Read the model definition and answer for the solid it produces. Units are mm, in the model's axes. Give positions to 0.01 mm unless a question says otherwise; leave off trailing zeros. Write each question's results on one line, items separated by ' | '. Start each with the question number.
Item 1: Determine the mould class of faces 1 (the cylindrical face through (-9.29, 3.13, 27.62)), 2 (the flat face through (0, 6.35, -1)), 3 (the cylindrical face through (-23.208, 3.219, 58.415)) for opening direction X: +X half, -X half, draft (parallel to the pull), parting line (faces both ways), or undercut.
Item 2: Section A-A on y = 4 is taken. State how many separate pieces and enclosed holes the cut face has, and give its area (3 significant figures).
Item 3: This flat-tipped pin is pushed along its axis until it touches: P1, Ø10, axis at x = 12.319, z = 28.575, coming from the +Y side. Where does it stop, or does it pass through?
Item 4: Find the intervals of material crossed by line 1 (X direction, y = 5.75, z = 49.5); line 2 (X direction, y = 5, z = -26); line 3 (Z direction, x = -22, y = 2.75), in increasing order.
```python
from build123d import *

# Parameters (mm, degrees)
SKETCH1_W           = 50.038
SKETCH1_H           = 120.65
SKETCH1_R           = 3.175
BOSS_EXTRUDE1_DEPTH = 6.35
FILLET1_R           = 6.35


with BuildPart() as part:
    # Sketch1 → Boss-Extrude1 (new body)
    with BuildSketch(Plane(origin=(0, 0, 0), x_dir=(1, 0, 0), z_dir=(0, 1, 0))):
        Rectangle(SKETCH1_W, SKETCH1_H)
        with Locations((12.319, -47.625)):
            Circle(SKETCH1_R, mode=Mode.SUBTRACT)
        with Locations((-12.319, -47.625)):
            Circle(SKETCH1_R, mode=Mode.SUBTRACT)
        with Locations((12.319, -28.575)):
            Circle(SKETCH1_R, mode=Mode.SUBTRACT)
        with Locations((-12.319, -28.575)):
            Circle(SKETCH1_R, mode=Mode.SUBTRACT)
        with Locations((12.319, -9.525)):
            Circle(SKETCH1_R, mode=Mode.SUBTRACT)
        with Locations((-12.319, -9.525)):
            Circle(SKETCH1_R, mode=Mode.SUBTRACT)
        with Locations((12.319, 9.525)):
            Circle(SKETCH1_R, mode=Mode.SUBTRACT)
        with Locations((-12.319, 9.525)):
            Circle(SKETCH1_R, mode=Mode.SUBTRACT)
        with Locations((12.319, 28.575)):
            Circle(SKETCH1_R, mode=Mode.SUBTRACT)
        with Locations((-12.319, 28.575)):
            Circle(SKETCH1_R, mode=Mode.SUBTRACT)
        with Locations((12.319, 47.625)):
            Circle(SKETCH1_R, mode=Mode.SUBTRACT)
        with Locations((-12.319, 47.625)):
            Circle(SKETCH1_R, mode=Mode.SUBTRACT)
    extrude(amount=BOSS_EXTRUDE1_DEPTH)

    # Fillet1
    fillet1_edges = [part.edges().sort_by_distance(p)[0] for p in [
        (25.019, 3.175, 60.325),
        (-25.019, 3.175, 60.325),
        (-25.019, 3.175, -60.325),
        (25.019, 3.175, -60.325),
    ]]
    fillet(fillet1_edges, radius=FILLET1_R)


solid = part.part
```
Findings:
1) face 1: undercut | face 2: draft | face 3: -X half
2) separate pieces: 1 | enclosed holes: 12 | area: 5,620 mm2
3) P1: y = 6.35
4) line 1: -25.02 to -14.88, -9.76 to 9.76, 14.88 to 25.02 | line 2: -25.02 to -14.18, -10.46 to 10.46, 14.18 to 25.02 | line 3: -59.38 to 59.38
